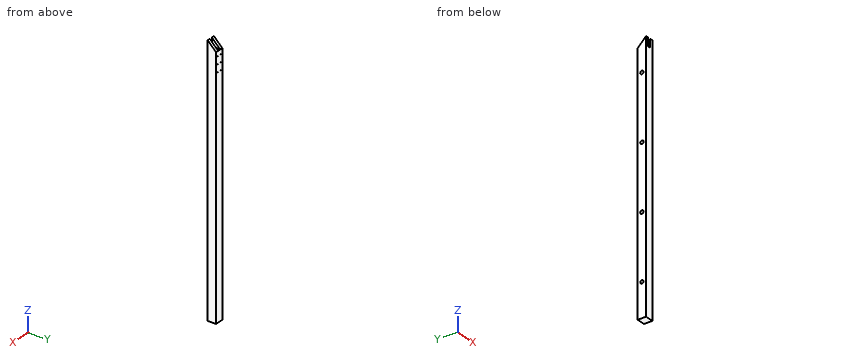
from build123d import *

# Parameters (mm, degrees)
F0_W     = 45
F0_H     = 1407
F1_DEPTH = 22.5
F3_SIZE2 = 44.99999
F3_SIZE  = 44.99999
F2_W     = 15
F2_H     = 45
F4_DEPTH = 45
F5_R     = 9
F6_DEPTH = 30
F9_D     = 3.5
F9_DEPTH = 30
F9_TIP   = 1.0515060833


# Not quite as in the source:
# - a fillet or chamfer is up to 0.001 mm smaller than in the source, because OpenCascade refuses the exact size


with BuildPart() as f1:
    # F0 (on Front) → F1 (new body, symmetric)
    with BuildSketch(Plane.XZ):
        with Locations((0, -490.1653682211)):
            Rectangle(F0_W, F0_H)
    extrude(amount=F1_DEPTH, both=True)

    # F3 (size 45 and 45 in the source; OpenCascade refuses exactly that, so slightly less here)
    f3_edges = [f1.edges().sort_by_distance(p)[0] for p in [
        (0, 22.5, 213.334632),
    ]]
    chamfer(f3_edges, length=F3_SIZE, length2=F3_SIZE2)

    # F2 (on face) → F4 (cut)
    with BuildSketch(Plane.XY.offset(213.3346317789)):
        Rectangle(F2_W, F2_H)
    extrude(amount=-F4_DEPTH, mode=Mode.SUBTRACT)

    # F5 (on face) → F6 (cut)
    with BuildSketch(Plane(origin=(-22.5, 0, 0), x_dir=(0, -1, 0), z_dir=(-1, 0, 0))):
        with Locations((0, 38.3346317789)):
            Circle(F5_R)
        with Locations((0, -311.6653682211)):
            Circle(F5_R)
        with Locations((0, -661.6653682211)):
            Circle(F5_R)
        with Locations((0, -1011.6653682211)):
            Circle(F5_R)
    extrude(amount=-F6_DEPTH, mode=Mode.SUBTRACT)

    # F9
    with Locations(Plane(origin=(0, 22.5, 0), x_dir=(-1, 0, 0), z_dir=(0, 1, 0))):
        with Locations((-10, 103.3346317789), (-10, 63.3346317789), (10, 63.3346317789), (10, 103.3346317789), (10, 143.3346317789), (-10, 143.3346317789)):
            Hole(F9_D / 2, depth=F9_DEPTH)
            with Locations((0, 0, -(F9_DEPTH + F9_TIP / 2))):  # 118° drill point
                Cone(0, F9_D / 2, F9_TIP, mode=Mode.SUBTRACT)


solid = f1.part
Input: part model. Units: mm. Frame: model coordinates. Coordinates: 2 decimals unless noted, no trailing zeros.
Q1. Material intervals for line 1 (Z direction, x = -19, y = -1.5); line 2 (Z direction, x = 0.5, y = 0); line 3 (Z direction, x = -10, y = 10), sorted ascending.
Q2. Cut plane A-A (y = -0.5). Give the number of separate pieces and of enclosed holes in the cut face, then the cut area to 3 significant figures.
Q3. Contact query for flat-ended pins moving along their axis: pin 1 (3 mm diameter, centred on x = -10, z = 63.33, fed in from +Y); pin 2 (16 mm diameter, centred on y = 0, z = 38.33, fed in from -X); pin 3 (8 mm diameter, centred on x = 7, y = 8.5, fed in from +Z); pin 4 (4.5 mm diameter, centred on x = 10, z = 103.33, fed in from +Y). Output: stop coordinate, or through.
Working result:
1. line 1: z = -1193.67 to -1020.54, -1002.79 to -670.54, -652.79 to -320.54, -302.79 to 29.46, 47.21 to 192.33
1. line 2: z = -1193.67 to -1020.67, -1002.67 to -670.67, -652.67 to -320.67, -302.67 to 29.33, 47.33 to 168.33
1. line 3: z = -1193.67 to 61.58, 65.08 to 101.58, 105.08 to 141.58, 145.08 to 180.83
2. separate pieces: 1
2. enclosed holes: 6
2. area: 59,800 mm2
3. pin 1: stops at y = -7.65
3. pin 2: stops at x = 7.5
3. pin 3: stops at z = 186.3
3. pin 4: stops at y = 22.5
